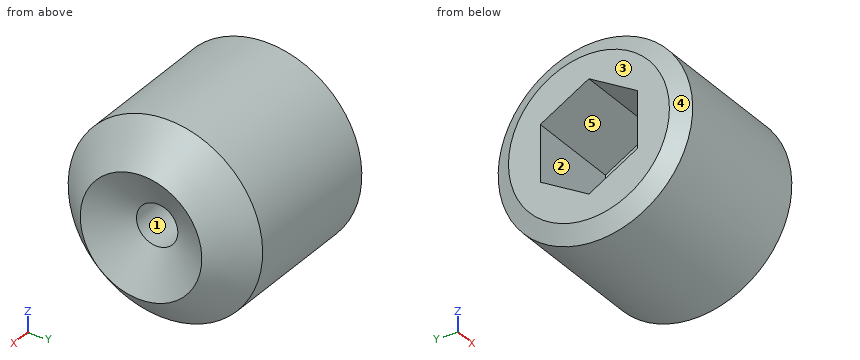
```python
from build123d import *

# Parameters (mm, degrees)
HEX_2_DEPTH        = 4
SKETCH6_R          = 0.85
CUT_EXTRUDE1_DEPTH = 10.797958971


with BuildPart() as part:
    # BodySke → BaseBody (revolve)
    with BuildSketch(Plane.XY, mode=Mode.PRIVATE) as basebody_sk:
        Polygon((0, 0), (0, 3.3095), (0.398660361, 4), (6.5, 4), (8, 2.5), (6.497848452, 0), align=None)
    revolve(basebody_sk.sketch.rotate(Axis((-12.7, 0, 0), (1, 0, 0)), 90), axis=Axis((-12.7, 0, 0), (1, 0, 0)))

    # Sketch2 → Hex 2 (cut)
    with BuildSketch(Plane.ZY):
        Polygon((1.154700538, 2), (-1.154700538, 2), (-2.309401077, 0), (-1.154700538, -2), (1.154700538, -2), (2.309401077, 0), align=None)
    extrude(amount=-HEX_2_DEPTH, mode=Mode.SUBTRACT)

    # Sketch6 → Cut-Extrude1 (cut, through all)
    with BuildSketch(Plane.ZY):
        with Locations(Location((0, 0, 0), (0, 0, 180))):
            Circle(SKETCH6_R)
    extrude(amount=-CUT_EXTRUDE1_DEPTH, mode=Mode.SUBTRACT)


solid = part.part
```
The model under review builds one solid part; all positions refer to its coordinate system, in mm. Face numbers are marked on the shaded views. A direction names the side the tool comes from. Round coordinates to 2 decimals unless told otherwise and drop trailing zeros. Write each loop counter-clockwise with the first axis right and the second up, starting at its lowest first coordinate (ties: lowest second). Pieces come first, ordered by that corner, then holes. Notation, with made-up numbers: M 57.25,78.25 L 86.25,78.25 A13 cw 86.25,101.25 Z; hole C -14.5,1.25 d10. An arc over 180 degrees is marked long. Use CSV: the item, a comma, the result in double quotes. Start each with the question number.
(1) The part is to be moulded in two halves that separate along Y. For the marked faces 3, 4 and 5, say which applies: +Y half, -Y half, draft (parallel to the pull), parting line (faces both ways), or undercut.
(2) Clearance check with flat-ended pins moving along their axes: P1, Ø4, axis at y = -2.5, z = -0.5, coming from the +X side; P2, Ø1.5, axis at y = 0, z = 0, coming from the +X side; P3, Ø3, axis at x = 1, z = -3, coming from the +Y side; P4, Ø2, axis at y = 0, z = 0, coming from the +X side. State where each tip first meets the part, or that it passes through.
(3) We need section B-B, the plane x = 1.25. State the section outline as (y, z) points, then the cut area to 3 significant figures.
(4) We need section C-C, the plane x = 6.75. State the section outline as (y, z) points.
(5) For line 1 along Y through (x, z) = (5.2, 0); line 2 along Y through (x, z) = (2.5, 0.25); line 3 along Z through (x, y) = (1.75, -1), list the stretches that pass through material, from the lowest coordinate up.
(6) Tool access review of the marked faces 1 and 2: name each direction out of +Z, -Z, +X, -X, +Y, -Y from which nothing blocks a thin tool from reaching the whole face with its end or side.
(7) We need section D-D, the plane x = 4.5. State the section outline as (y, z) points.
(8) We need section A-A, the plane z = 0. State the section outline as (x, y) points, then the cut area to 3 significant figures.
Findings:
1,face 3,"draft"
1,face 4,"parting line"
1,face 5,"undercut"
2,P1,"x = 8"
2,P2,"through"
2,P3,"y = 3.71"
2,P4,"x = 7.1"
3,outline,"C 0,0 d8; hole M -2,-1.15 L 0,-2.31 L 2,-1.15 L 2,1.15 L 0,2.31 L -2,1.15 Z"
3,area,"36.4 mm^2"
4,outline,"C 0,0 d7.5; hole C 0,0 d1.7"
5,line 1,"-4 to -0.85, 0.85 to 4"
5,line 2,"-3.99 to -2, 2 to 3.99"
5,line 3,"-3.87 to -1.73, 1.73 to 3.87"
6,face 1,"+X, -X"
6,face 2,"-X"
7,outline,"C 0,0 d8; hole C 0,0 d1.7"
8,outline,"M 0,-3.31 L 0.4,-4 L 6.5,-4 L 8,-2.5 L 7.01,-0.85 L 4,-0.85 L 4,-2 L 0,-2 Z; M 0,2 L 4,2 L 4,0.85 L 7.01,0.85 L 8,2.5 L 6.5,4 L 0.4,4 L 0,3.31 Z"
8,area,"37.0 mm^2"
